from build123d import *

# Parameters (mm, degrees)
SKETCH1_W            = 1220
SKETCH1_H            = 915
BOSS_EXTRUDE1_DEPTH  = 254
SHELL1_T             = -7
BOSS_EXTRUDE2_DEPTH  = 901
SKETCH3_W            = 175
SKETCH3_H            = 185
SKETCH3_W_2          = 165
SKETCH3_H_2          = 175
BOSS_EXTRUDE3_DEPTH  = 135
BOSS_EXTRUDE4_DEPTH  = 175
BOSS_EXTRUDE5_DEPTH  = 5
BOSS_EXTRUDE6_DEPTH  = 5
SKETCH7_W            = 1220
SKETCH7_H            = 7
BOSS_EXTRUDE7_DEPTH  = 320
SKETCH8_W            = 1348.114973262
SKETCH8_H            = 350.584679525
CUT_EXTRUDE1_DEPTH   = 8
SKETCH9_R            = 7
CUT_EXTRUDE2_DEPTH   = 10
SKETCH10_W           = 1220
SKETCH10_H           = 230
BOSS_EXTRUDE8_DEPTH  = 10
SKETCH12_W           = 1206
SKETCH12_H           = 223
BOSS_EXTRUDE10_DEPTH = 10
SKETCH14_W           = 13.994838931
SKETCH14_H           = 66.246220617
BOSS_EXTRUDE13_DEPTH = 1219.2
SKETCH15_W           = 1075.77038164
SKETCH15_H           = 47.733443392
CUT_EXTRUDE3_DEPTH   = 10
SKETCH16_R           = 11.892366701
CUT_EXTRUDE4_DEPTH   = 10


with BuildPart() as part:
    # Sketch1 → Boss-Extrude1 (new body)
    with BuildSketch(Plane(origin=(0, 0, 0), x_dir=(1, 0, 0), z_dir=(0, 1, 0))):
        Rectangle(SKETCH1_W, SKETCH1_H)
    extrude(amount=BOSS_EXTRUDE1_DEPTH)

    # Shell1
    shell1_openings = [part.faces().sort_by_distance(p)[0] for p in [
        (0, 254, 0),
    ]]
    offset(amount=SHELL1_T, openings=shell1_openings, kind=Kind.INTERSECTION)

    # Sketch2 → Boss-Extrude2 (add)
    with BuildSketch(Plane.XY.offset(-450.5)):
        Polygon((-87.5, 164.514526371), (-603, 194.514526371), (-603, 186.514526371), (-87.5, 156.514526371), align=None)
        Polygon((603, 194), (87.5, 164.514526371), (87.5, 156.514526371), (603, 186), align=None)
    extrude(amount=BOSS_EXTRUDE2_DEPTH)

    # Sketch3 → Boss-Extrude3 (add)
    with BuildSketch(Plane(origin=(0, 7, 0), x_dir=(1, 0, 0), z_dir=(0, 1, 0))):
        Rectangle(SKETCH3_W, SKETCH3_H)
        Rectangle(SKETCH3_W_2, SKETCH3_H_2, mode=Mode.SUBTRACT)
    extrude(amount=BOSS_EXTRUDE3_DEPTH)

    # Sketch4 → Boss-Extrude4 (add)
    with BuildSketch(Plane.ZY.offset(-87.5)):
        Polygon((92.5, 142), (450.5, 156.514526371), (450.5, 151.514526371), (92.5, 137), align=None)
        Polygon((-92.5, 142), (-450.5, 156.514526371), (-450.5, 151.514526371), (-92.5, 137), align=None)
    extrude(amount=BOSS_EXTRUDE4_DEPTH)

    # Sketch5 → Boss-Extrude5 (add)
    with BuildSketch(Plane(origin=(-87.5, 0, 0), x_dir=(0, 0, -1), z_dir=(1, 0, 0))):
        Polygon((450.5, 164.514526371), (450.5, 156.514526371), (92.5, 142), (-92.5, 142), (-450.5, 156.514526371), (-450.5, 164.514526371), align=None)
    extrude(amount=BOSS_EXTRUDE5_DEPTH)

    # Sketch6 → Boss-Extrude6 (add)
    with BuildSketch(Plane.ZY.offset(-87.5)):
        Polygon((450.5, 164.514526371), (450.5, 156.514526371), (92.5, 142), (-92.5, 142), (-450.5, 156.514526371), (-450.5, 164.514526371), align=None)
    extrude(amount=BOSS_EXTRUDE6_DEPTH)

    # Sketch7 → Boss-Extrude7 (add)
    with BuildSketch(Plane(origin=(0, 254, 0), x_dir=(1, 0, 0), z_dir=(0, 1, 0))):
        with Locations((0, -454)):
            Rectangle(SKETCH7_W, SKETCH7_H)
    extrude(amount=BOSS_EXTRUDE7_DEPTH)

    # Sketch8 → Cut-Extrude1 (cut, through all)
    with BuildSketch(Plane(origin=(0, 0, 450.5), x_dir=(-1, 0, 0), z_dir=(0, 0, -1))):
        with Locations((-20.633408071, 430.569613213)):
            Rectangle(SKETCH8_W, SKETCH8_H)
    extrude(amount=-CUT_EXTRUDE1_DEPTH, mode=Mode.SUBTRACT)

    # Sketch9 → Cut-Extrude2 (cut)
    with BuildSketch(Plane.XY.offset(457.5)):
        with Locations((0, 34)):
            Circle(SKETCH9_R)
    extrude(amount=-CUT_EXTRUDE2_DEPTH, mode=Mode.SUBTRACT)

    # Sketch10 → Boss-Extrude8 (add)
    with BuildSketch(Plane(origin=(0, 254, 0), x_dir=(1, 0, 0), z_dir=(0, 1, 0))):
        with Locations((0, -342.5)):
            Rectangle(SKETCH10_W, SKETCH10_H)
    extrude(amount=BOSS_EXTRUDE8_DEPTH)

    # Sketch12 → Boss-Extrude10 (add)
    with BuildSketch(Plane(origin=(0, 199, 0), x_dir=(-1, 0, 0), z_dir=(0, -1, 0))):
        with Locations((0, -339)):
            Rectangle(SKETCH12_W, SKETCH12_H)
    extrude(amount=-BOSS_EXTRUDE10_DEPTH)

    # Sketch14 → Boss-Extrude13 (add)
    with BuildSketch(Plane(origin=(610, 0, 0), x_dir=(0, 0, -1), z_dir=(1, 0, 0))):
        with Locations((-222.206337189, 230.567579207)):
            Rectangle(SKETCH14_W, SKETCH14_H)
    extrude(amount=-BOSS_EXTRUDE13_DEPTH)

    # Sketch15 → Cut-Extrude3 (cut)
    with BuildSketch(Plane(origin=(0, 264, 0), x_dir=(1, 0, 0), z_dir=(0, 1, 0))):
        with Locations((3.093834294, -328.830387814)):
            Rectangle(SKETCH15_W, SKETCH15_H)
    extrude(amount=-CUT_EXTRUDE3_DEPTH, mode=Mode.SUBTRACT)

    # Sketch16 → Cut-Extrude4 (cut)
    with BuildSketch(Plane.XY.offset(457.5)):
        with Locations((0, 177.972608665)):
            Circle(SKETCH16_R)
    extrude(amount=-CUT_EXTRUDE4_DEPTH, mode=Mode.SUBTRACT)


solid = part.part
Can you work these out from the model? Positions are in its coordinate system, mm. A direction names the side the tool comes from. Give positions to 0.01 mm unless a question says otherwise; leave off trailing zeros. Order: outer loops, then holes, each group sorted by start corner. A loop starts at its lowest first (then second) coordinate and runs counter-clockwise, first axis right, second up. Notation, with made-up numbers: M 20.5,7.25 L 51.5,7.25 A23 cw 51.5,41.25 Z; hole C -12.75,8.5 d4. An arc over 180 degrees is marked long. Use one line per item in the form item = value. Start each with the question number.
Item 1: If we section it at C-C (x = -387): Write out the boundary of the cut face in (y, z).
Item 2: If I drill on line 1 along Y through (x, z) = (0, 453); line 2 along Z through (x, y) = (423, 198); line 3 along Z through (x, y) = (23, 51), over which ranges is the centre line in solid material (lowest first)?
Item 3: If we section it at D-D (z = -65.5): Write out the boundary of the cut face in (x, y), then the cut area to 3 significant figures.
Item 4: Will these pins go through, and if not, where does the flat tip stop? pin 1 Ø4 at (x, z) = (261.5, 249.5) entering from -Y; pin 2 Ø3 at (x, y) = (182.5, 259.5) entering from -Z.
Item 5: If we section it at A-A (y = 53.5): Write out the boundary of the cut face in (x, z).
Item 6: For faces 5 (the flat face through (-603, 96, 6)), 6 (the flat face through (-1, 7, -1)), 7 (the flat face through (-610, 130, 6)), which set-ups out of +Z, -Z, +X, -X, +Y, -Y let a thin tool reach every point of the face, with its end or its side?
Item 7: If we section it at B-B (z = -366): Write out the boundary of the cut face in (x, y), then the cut area to 3 significant figures.
Item 8: We'd pull the mould along Y, two halves only. Please class faces 1 (the flat face through (1.22, 144.36, -274.01)), 2 (the flat face through (1.155, 149.156, -268.994)), 3 (the flat face through (610, 130, 6)), 4 (the flat face through (87.5, 99, 2)): +Y half, -Y half, draft (parallel to the pull), parting line (faces both ways), or undercut.
Outcome:
q1.outline = M 0,-457.5 L 254,-457.5 L 254,-450.5 L 181.94,-450.5 L 181.94,450.5 L 199,450.5 L 199,229.2 L 197.44,229.2 L 197.44,215.21 L 263.69,215.21 L 263.69,227.5 L 264,227.5 L 264,304.96 L 254,304.96 L 254,229.2 L 209,229.2 L 209,450.5 L 254,450.5 L 254,352.7 L 264,352.7 L 264,457.5 L 0,457.5 Z; hole M 7,-450.5 L 173.94,-450.5 L 173.94,450.5 L 7,450.5 Z
q2.line_1 = 0 to 27, 41 to 166.08, 189.86 to 264
q2.line_2 = -457.5 to -450.5, 215.21 to 229.2, 450.5 to 457.5
q2.line_3 = -457.5 to -450.5, -92.5 to -87.5, 87.5 to 92.5, 450.5 to 457.5
q3.outline = M -610,0 L 610,0 L 610,254 L 603,254 L 603,194 L 87.5,164.51 L 82.5,164.51 L 82.5,7 L -82.5,7 L -82.5,164.51 L -87.5,164.51 L -603,194.51 L -603,254 L -610,254 Z; hole M -603,7 L -87.5,7 L -87.5,156.51 L -603,186.51 Z; hole M 87.5,7 L 603,7 L 603,186 L 87.5,156.51 Z
q3.area = 21,800 mm2
q4.pin_1 = 0
q4.pin_2 = 215.21
q5.outline = M -610,-457.5 L 610,-457.5 L 610,457.5 L -610,457.5 Z; M -87.5,-92.5 L 87.5,-92.5 L 87.5,92.5 L -87.5,92.5 Z; hole M -603,-450.5 L 603,-450.5 L 603,450.5 L -603,450.5 Z; hole M -82.5,-87.5 L 82.5,-87.5 L 82.5,87.5 L -82.5,87.5 Z
q6.face_5 = none
q6.face_6 = +Y
q6.face_7 = +Z, -Z, -X, +Y, -Y
q7.outline = M -610,0 L 610,0 L 610,254 L 603,254 L 603,194 L 87.5,164.51 L 82.5,164.51 L 82.5,153.09 L -82.5,153.09 L -82.5,164.51 L -87.5,164.51 L -603,194.51 L -603,254 L -610,254 Z; hole M -603,7 L 603,7 L 603,186 L 87.5,156.51 L 87.5,148.09 L -87.5,148.09 L -87.5,156.51 L -603,186.51 Z
q7.area = 21,200 mm2
q8.face_1 = undercut
q8.face_2 = +Y half
q8.face_3 = draft
q8.face_4 = undercut
